Input: part model. Units: mm. Frame: model coordinates. A direction names the side the tool comes from. Coordinates: 2 decimals unless noted, no trailing zeros. Loops run counter-clockwise (first coordinate to the right, second up) from the corner with the lowest first, then second, coordinate; pieces in that order, holes last. Notation, with made-up numbers: (-34, 37) -> (-19, 37) arc R15 cw to (-19, 58) -> close; hole circle Ø11 at (85, 70). An arc over 180 degrees is marked (long way). Answer as a JSON object with one key per item and string values.
from build123d import *

# Parameters (mm, degrees)
SKETCH2_R          = 2.75
CUT_EXTRUDE1_DEPTH = 10


with BuildPart() as part:
    # Sketch1 → Revolve1 (revolve)
    with BuildSketch(Plane.XY, mode=Mode.PRIVATE) as revolve1_sk:
        Polygon((10, 0), (10, 6), (44, 6), (44, 13), (34, 13), (34, 14), (10, 14), (10, 13), (0, 13), (0, 0), align=None)
    revolve(revolve1_sk.sketch.rotate(Axis((0, 24, 0), (1, 0, 0)), 270), axis=Axis((0, 24, 0), (1, 0, 0)))

    # Sketch2 → Cut-Extrude1 (cut)
    with BuildSketch(Plane.ZY):
        with Locations((0, 42.971966769)):
            Circle(SKETCH2_R)
        with Locations((16.454482672, 33.471966769)):
            Circle(SKETCH2_R)
        with Locations((16.454482672, 14.471966769)):
            Circle(SKETCH2_R)
        with Locations((0, 4.971966769)):
            Circle(SKETCH2_R)
        with Locations((-16.454482672, 14.471966769)):
            Circle(SKETCH2_R)
        with Locations((-16.454482672, 33.471966769)):
            Circle(SKETCH2_R)
    extrude(amount=-CUT_EXTRUDE1_DEPTH, mode=Mode.SUBTRACT)


solid = part.part
1. Line query: line 1 along Y through (x, z) = (4.5, 0); line 2 along Y through (x, z) = (22.5, -3); line 3 along Z through (x, y) = (8, 45). Output: solid intervals per line, ascending.
Reply:
{"line 1": "y = 0 to 2.22, 7.72 to 13, 35 to 40.22, 45.72 to 48", "line 2": "y = 6.25 to 14.46, 33.54 to 41.75", "line 3": "z = -11.62 to -1.86, 1.86 to 11.62"}
2. Access query for faces 1 (the face through (10, 6, -4)), 2 (the face through (0, 34, -5)), 3 (the face through (4.9, 17.2, -16.8)). Directions: +Z, -Z, +X, -X, +Y, -Y. A direction counts if a zero-diameter tool reaches every point of the face in a straight line with its end or side. Return the directions, or none.
Reply:
{"face 1": "+X", "face 2": "+Z, -Z, -X, +Y, -Y", "face 3": "-X"}
3. Section query B-B (z = 0). Return loops of the section in (x, y).
Reply:
{"outline": "(0, 0) -> (10, 0) -> (10, 2.22) -> (0, 2.22) -> close; (0, 7.72) -> (10, 7.72) -> (10, 6) -> (44, 6) -> (44, 13) -> (34, 13) -> (34, 14) -> (10, 14) -> (10, 13) -> (0, 13) -> close; (0, 35) -> (10, 35) -> (10, 34) -> (34, 34) -> (34, 35) -> (44, 35) -> (44, 42) -> (10, 42) -> (10, 40.22) -> (0, 40.22) -> close; (0, 45.72) -> (10, 45.72) -> (10, 48) -> (0, 48) -> close"}
4. Section query A-A (y = 24). Return loops of the section in (x, z), plus the area to 3 significant figures.
Reply:
{"outline": "(0, -24) -> (10, -24) -> (10, -18) -> (44, -18) -> (44, -11) -> (34, -11) -> (34, -10) -> (10, -10) -> (10, -11) -> (0, -11) -> close; (0, 11) -> (10, 11) -> (10, 10) -> (34, 10) -> (34, 11) -> (44, 11) -> (44, 18) -> (10, 18) -> (10, 24) -> (0, 24) -> close", "area": "784 mm2"}
5. Pin query (flat end, axial travel): P1, Ø0.9, axis at y = 7, z = 0.5, coming from the -X side; P2, Ø1.5, axis at x = 29.5, y = 17.5, coming from the +Z side; P3, Ø4, axis at x = 36.5, y = 13.5, coming from the -Z side. Return the tip coordinate at first contact, or that it passes through.
Reply:
{"P1": "stops at x = 10", "P2": "stops at z = 17.06", "P3": "stops at z = -15.87"}
6. Section query C-C (z = -16). Return loops of the section in (x, y), plus the area to 3 significant figures.
Reply:
{"outline": "(0, 6.11) -> (10, 6.11) -> (10, 11.76) -> (0, 11.76) -> close; (0, 17.18) -> (10, 17.18) -> (10, 15.75) -> (44, 15.75) -> (44, 32.25) -> (10, 32.25) -> (10, 30.76) -> (0, 30.76) -> close; (0, 36.18) -> (10, 36.18) -> (10, 41.89) -> (0, 41.89) -> close", "area": "810 mm2"}
7. Mould query, pull axis Y, two halves, no side actions, for faces 4 (the face through (5.07, 33.19, 22.17)), 5 (the face through (44, 32, -8)), 6 (the face through (4.93, 16.791, 17.933)). Classes: pulls with the +Y half, pulls with the -Y half, needs draft (parallel to the pull), parting line crosses it, or undercut.
Reply:
{"face 4": "parting line crosses it", "face 5": "needs draft", "face 6": "undercut"}
8. Section query D-D (x = 40). Return loops of the section in (y, z), plus the area to 3 significant figures.
Reply:
{"outline": "circle Ø36 at (24, 0); hole circle Ø22 at (24, 0)", "area": "638 mm2"}
